Model file for the job. Use its own axes, mm. A direction names the side the tool comes from. Coordinates: 2 decimals unless noted, no trailing zeros. Order: outer loops, then holes, each group sorted by start corner. A loop starts at its lowest first (then second) coordinate and runs counter-clockwise, first axis right, second up.
from build123d import *

# Parameters (mm, degrees)
BOSS_EXTRUDE1_DEPTH = 114.3
SHELL1_T            = -12.7
CUT_EXTRUDE1_DEPTH  = 222.690489912
FILLET1_R           = 48.26
FILLET2_R           = 48.26


with BuildPart() as part:
    # Sketch2 → Boss-Extrude1 (new body)
    with BuildSketch(Plane(origin=(0, 0, 0), x_dir=(1, 0, 0), z_dir=(0, 1, 0))):
        with BuildLine():
            Line((-127, 101.6), (-127, -101.6))
            ThreePointArc((-127, -101.6), (-125.402452129, -121.680463142), (-120.65, -141.25573729))
            Line((-120.65, -141.25573729), (120.65, -141.25573729))
            ThreePointArc((120.65, -141.25573729), (125.402452129, -121.680463142), (127, -101.6))
            Line((127, -101.6), (127, 101.6))
            ThreePointArc((127, 101.6), (125.402452129, 121.680463142), (120.65, 141.25573729))
            Line((120.65, 141.25573729), (-120.65, 141.25573729))
            ThreePointArc((-120.65, 141.25573729), (-125.402452129, 121.680463142), (-127, 101.6))
        make_face()
    extrude(amount=BOSS_EXTRUDE1_DEPTH)

    # Shell1
    shell1_openings = [part.faces().sort_by_distance(p)[0] for p in [
        (0, 114.3, 0),
    ]]
    offset(amount=SHELL1_T, openings=shell1_openings, kind=Kind.INTERSECTION)

    # Sketch3 → Cut-Extrude1 (cut, through all)
    # profile 1 of 2: a face of its own
    with BuildSketch(Plane.XY):
        with BuildLine():
            Line((-72.268980264, 88.9), (72.268980264, 88.9))
            ThreePointArc((72.268980264, 88.9), (104.018980264, 57.15), (72.268980264, 25.4))
            Line((72.268980264, 25.4), (-72.268980264, 25.4))
            ThreePointArc((-72.268980264, 25.4), (-104.018980264, 57.15), (-72.268980264, 88.9))
        make_face()
        with BuildLine():
            ThreePointArc((72.268980264, 31.75), (97.668980264, 57.15), (72.268980264, 82.55))
            Line((72.268980264, 82.55), (-72.268980264, 82.55))
            ThreePointArc((-72.268980264, 82.55), (-97.668980264, 57.15), (-72.268980264, 31.75))
            Line((-72.268980264, 31.75), (72.268980264, 31.75))
        make_face(mode=Mode.SUBTRACT)
    # profile 2 of 2: a face of its own
    with BuildSketch(Plane.XY):
        with BuildLine():
            Line((-72.268980264, 31.75), (72.268980264, 31.75))
            ThreePointArc((72.268980264, 31.75), (97.668980264, 57.15), (72.268980264, 82.55))
            Line((72.268980264, 82.55), (-72.268980264, 82.55))
            ThreePointArc((-72.268980264, 82.55), (-97.668980264, 57.15), (-72.268980264, 31.75))
        make_face()
    extrude(amount=-CUT_EXTRUDE1_DEPTH, mode=Mode.SUBTRACT)

    # Fillet1
    fillet1_edges = [part.edges().sort_by_distance(p)[0] for p in [
        (120.65, 57.15, 141.25573729),
        (-120.65, 57.15, 141.25573729),
    ]]
    fillet(fillet1_edges, radius=FILLET1_R)

    # Fillet2
    # the kernel refuses this fillet: 48.26 mm, written as the material it takes off along each edge
    with BuildSketch(Plane(origin=(-120.65, -121.689926144, -141.25573729), x_dir=(-0.13045451257138782, 0, 0.9914542955425437), z_dir=(0, 1, 0))) as fillet2_piece_1:
        with BuildLine():
            CenterArc((42.380235681, 47.847584303), FILLET2_R, 187.49585764, 90)
            Line((-5.467348622, 41.551849526), (-10.252107052, 40.922276049))
            Line((-10.252107052, 40.922276049), (-4.78475843, -0.629573478))
            Line((-4.78475843, -0.629573478), (-0.895945537, -4.742104764))
            ThreePointArc((-0.895945537, -4.742104764), (40.774810711, -5.907223328), (49.305543935, -4.78475843))
            Line((49.305543935, -4.78475843), (48.675970458, 0))
        make_face()
    extrude(amount=357.679852289, mode=Mode.SUBTRACT)
    with BuildSketch(Plane(origin=(120.65, -121.689926144, -141.25573729), x_dir=(-1, 0, 0), z_dir=(0, 1, 0))) as fillet2_piece_2:
        with BuildLine():
            CenterArc((41.91, 48.26), FILLET2_R, 180, 90)
            Line((-6.35, 48.26), (-11.176, 48.26))
            ThreePointArc((-11.176, 48.26), (-11.176, 39.65573729), (-4.5847, -1.506918017))
            Line((-4.5847, -1.506918017), (0, -4.826))
            Line((0, -4.826), (41.91, -4.826))
            Line((41.91, -4.826), (41.91, 0))
        make_face()
    extrude(amount=357.679852289, mode=Mode.SUBTRACT)


solid = part.part
Q1. Cut at B-B, the plane z = -74.5. List the corners of the cut face in (x, y), plus the area to 3 significant figures.
Established:
outline: (-127, 0) - (127, 0) - (127, 114.3) - (114.3, 114.3) - (114.3, 12.7) - (-114.3, 12.7) - (-114.3, 114.3) - (-127, 114.3) - close
area: 5,810 mm2
Q2. Mould opens along Z. For faces 1 (the face through (118.6, 56.3, -120.2)), 2 (the face through (-127, 56, -1)), 3 (the face through (114.3, 63, 1)) say: pulls with the +Z half, pulls with the -Z half, needs draft (parallel to the pull), parting line crosses it, or undercut.
Established:
face 1: pulls with the -Z half
face 2: needs draft
face 3: undercut
Q3. Probe line 1 (X direction, y = 48, z = 66); line 2 (Z direction, x = 68, y = 91); line 3 (Y direction, x = -0.5, z = -88). List the from-to ranges inside material, lowest first.
Established:
line 1: x = -127 to -114.3, 114.3 to 127
line 2: z = -141.26 to -128.56, 128.56 to 141.26
line 3: y = 0 to 12.7
Q4. Cut at A-A, the plane x = 69. List the corners of the cut face in (y, z).
Established:
outline: (0, -141.26) - (25.4, -141.26) - (25.4, -128.56) - (12.7, -128.56) - (12.7, 128.56) - (114.3, 128.56) - (114.3, 141.26) - (0, 141.26) - close; (88.9, -141.26) - (114.3, -141.26) - (114.3, -128.56) - (88.9, -128.56) - close
Q5. Cut at C-C, the plane z = -124. List the corners of the cut face in (x, y), plus the area to 3 significant figures.
Established:
outline: (-115.72, 0) - (115.72, 0) - (115.72, 114.3) - (112.08, 114.3) - (112.08, 12.7) - (-112.08, 12.7) - (-112.08, 114.3) - (-115.72, 114.3) - close
area: 3,680 mm2
Q6. Which spindle directions (+Z, -Z, +X, -X, +Y, -Y) get a long thin tool onto all of the face, cutting with end or side? Do faces 4 (the face through (1, 25.4, -135)), 5 (the face through (-113.514, 62.789, 114.985)), 6 (the face through (-1, 56, 141.256)). Say none if no direction does.
Established:
face 4: -Z
face 5: +Y
face 6: +Z, +X, -X, +Y, -Y
Q7. Drop flat-ended pins along their axis: P1, Ø4, axis at x = -87, y = 64, coming from the +Z side; P2, Ø4, axis at y = 58.5, z = 107, coming from the +X side; P3, Ø1.5, axis at x = -16.5, y = 34, coming from the -Z side. Give the stop position or say it passes through.
Established:
P1: stops at z = 140.85
P2: stops at x = 125.48
P3: stops at z = 128.56
